For this review, use the dimensioned drawing (mm, ordinates from the lowest corner) and the shaded views. Round coordinates to 2 decimals unless told otherwise and drop trailing zeros. Write each loop counter-clockwise with the first axis right and the second up, starting at its lowest first coordinate (ties: lowest second). Pieces come first, ordered by that corner, then holes. Notation, with made-up numbers: (-39.75, 61) -> (-15.75, 61) arc R25 ccw to (-15.75, 98) -> close; hole circle Ø2 at (44.5, 82). An arc over 180 degrees is marked (long way). Write each question's results on one line, items separated by ' | '. Start each with the question number.
Item 1: Add section C-C (x = 34). State the section outline as (y, z) points, plus the area to 3 significant figures.
Item 2: To check wall thickness, follow line 1 along Y through (x, z) = (30.5, 2.95); line 2 along Z through (x, y) = (14, 4.1); line 3 along Y through (x, z) = (27, 3.7). State the ranges of each line that lie inside material, in increasing order.
Item 3: Add section A-A (y = 3). State the section outline as (x, z) points, plus the area to 3 significant figures.
Item 4: Add section D-D (z = 5.55). State the section outline as (x, y) points.
Item 5: Clearance check with flat-ended pins moving along their axes: pin 1 (1 mm diameter, centred on x = 22.5, y = 2, fed in from +Z); pin 2 (1 mm diameter, centred on x = 17, y = 4, fed in from -Z). State where each tip first meets the part, or that it passes through.
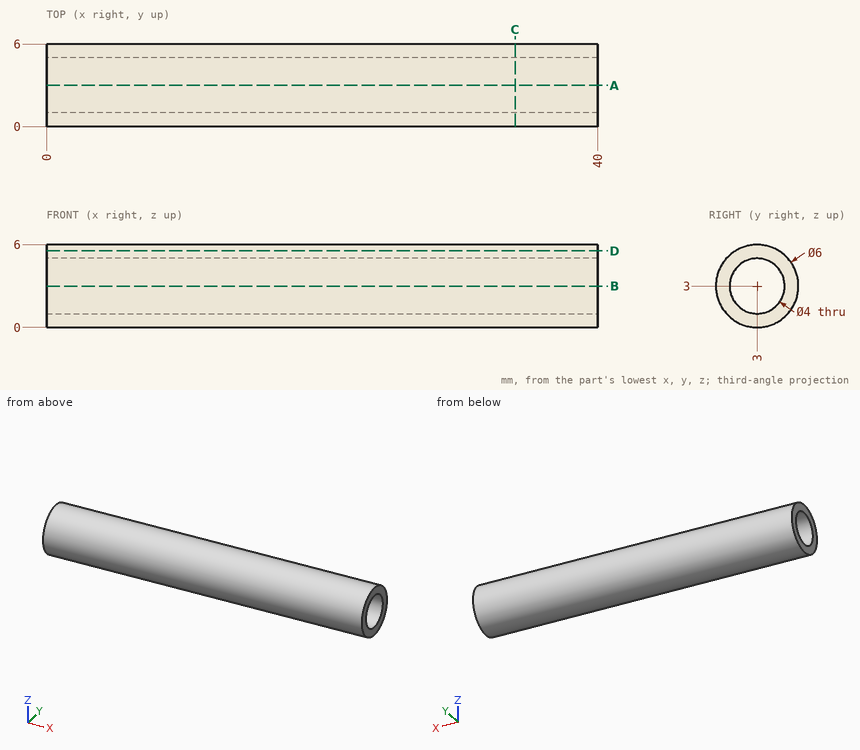
Responses:
1) outline: circle Ø6 at (3, 3); hole circle Ø4 at (3, 3) | area: 15.7 mm^2
2) line 1: y = 0 to 1, 5 to 6 | line 2: z = 0.21 to 1.33, 4.67 to 5.79 | line 3: y = 0.08 to 1.13, 4.87 to 5.92
3) outline: (0, 0) -> (40, 0) -> (40, 1) -> (0, 1) -> close; (0, 5) -> (40, 5) -> (40, 6) -> (0, 6) -> close | area: 80.0 mm^2
4) outline: (0, 1.42) -> (40, 1.42) -> (40, 4.58) -> (0, 4.58) -> close
5) pin 1: stops at z = 5.96 | pin 2: stops at z = 0.04
